Autodesk Fusion 360 part; units mm, degrees
sketch "스케치1" plane through (0, 0, 0) normal (0, 1, 0) x (1, 0, 0)
  line L0 (10, -10) -> (-10, -10)
  line L1 (-10, -10) -> (-10, 10)
  line L2 (-10, 10) -> (10, 10)
  line L3 (10, 10) -> (10, -10)
  line L4 (10, -10) -> (-10, 10) construction
  line L5 (-10, -10) -> (10, 10) construction
  line L6 (10, 0) -> (10, -4.15)
  line L7 (3.3, 0) -> (3.3, 4.15)
  line L8 (3.3, 4.15) -> (10, 4.15)
  line L9 (10, 4.15) -> (10, -4.15)
  line L10 (10, -4.15) -> (3.3, -4.15)
  line L11 (3.3, -4.15) -> (3.3, 4.15)
  line L12 (10, -4.15) -> (8.5, -4.15)
  line L13 (8.5, -4.15) -> (8.5, -2.65)
  line L14 (8.5, -2.65) -> (10, -2.65)
  line L15 (10, -2.65) -> (10, -4.15)
  line L16 (10, 4.15) -> (8.5, 4.15)
  line L17 (8.5, 4.15) -> (8.5, 2.65)
  line L18 (8.5, 2.65) -> (10, 2.65)
  line L19 (10, 2.65) -> (10, 4.15)
  line L20 (8.5, 4.15) -> (5.5, 4.15)
  line L21 (5.5, 4.15) -> (5.5, -4.15)
  line L22 (5.5, -4.15) -> (8.5, -4.15)
  line L23 (8.5, -4.15) -> (8.5, 4.15)
  spline S0 degree 5 poles (5.5, -4.15) (5.3331, -3.984) (5.014, -3.652) (4.579, -3.154) (4.0878, -2.49) (3.6321, -1.66) (3.3486, -0.83) (3.2516, 0) (3.3486, 0.83) (3.6321, 1.66) (4.0878, 2.49) (4.579, 3.154) (5.014, 3.652) (5.3331, 3.984) (5.5, 4.15) knots 0 0 0 0 0 0 0.1 0.2 0.3 0.4 0.5 0.6 0.7 0.8 0.9 1 1 1 1 1 1
  spline S1 degree 5 poles (4.15, 5.5) (3.984, 5.3331) (3.652, 5.014) (3.154, 4.579) (2.49, 4.0878) (1.66, 3.6321) (0.83, 3.3486) (0, 3.2516) (-0.83, 3.3486) (-1.66, 3.6321) (-2.49, 4.0878) (-3.154, 4.579) (-3.652, 5.014) (-3.984, 5.3331) (-4.15, 5.5) knots 0 0 0 0 0 0 0.1 0.2 0.3 0.4 0.5 0.6 0.7 0.8 0.9 1 1 1 1 1 1
  line L24 (4.15, 5.5) -> (4.15, 8.5)
  line L25 (4.15, 8.5) -> (2.65, 8.5)
  line L26 (2.65, 8.5) -> (2.65, 10)
  line L27 (-4.15, 8.5) -> (-4.15, 5.5)
  line L28 (-4.15, 8.5) -> (-2.65, 8.5)
  line L29 (-2.65, 8.5) -> (-2.65, 10)
  spline S2 degree 5 poles (-5.5, 4.15) (-5.3331, 3.984) (-5.014, 3.652) (-4.579, 3.154) (-4.0878, 2.49) (-3.6321, 1.66) (-3.3486, 0.83) (-3.2516, 0) (-3.3486, -0.83) (-3.6321, -1.66) (-4.0878, -2.49) (-4.579, -3.154) (-5.014, -3.652) (-5.3331, -3.984) (-5.5, -4.15) knots 0 0 0 0 0 0 0.1 0.2 0.3 0.4 0.5 0.6 0.7 0.8 0.9 1 1 1 1 1 1
  line L30 (-5.5, 4.15) -> (-8.5, 4.15)
  line L31 (-8.5, 4.15) -> (-8.5, 2.65)
  line L32 (-8.5, 2.65) -> (-10, 2.65)
  line L33 (-8.5, -4.15) -> (-5.5, -4.15)
  line L34 (-8.5, -4.15) -> (-8.5, -2.65)
  line L35 (-8.5, -2.65) -> (-10, -2.65)
  spline S3 degree 5 poles (-4.15, -5.5) (-3.984, -5.3331) (-3.652, -5.014) (-3.154, -4.579) (-2.49, -4.0878) (-1.66, -3.6321) (-0.83, -3.3486) (0, -3.2516) (0.83, -3.3486) (1.66, -3.6321) (2.49, -4.0878) (3.154, -4.579) (3.652, -5.014) (3.984, -5.3331) (4.15, -5.5) knots 0 0 0 0 0 0 0.1 0.2 0.3 0.4 0.5 0.6 0.7 0.8 0.9 1 1 1 1 1 1
  line L36 (-4.15, -5.5) -> (-4.15, -8.5)
  line L37 (-4.15, -8.5) -> (-2.65, -8.5)
  line L38 (-2.65, -8.5) -> (-2.65, -10)
  line L39 (4.15, -8.5) -> (4.15, -5.5)
  line L40 (4.15, -8.5) -> (2.65, -8.5)
  line L41 (2.65, -8.5) -> (2.65, -10)
  line L42 (-10, -10) -> (-4.15, -10)
  line L43 (-4.15, -10) -> (-4.15, -4.15)
  line L44 (-4.15, -4.15) -> (-10, -4.15)
  line L45 (-10, -4.15) -> (-10, -10)
  circle A0 centre (-7.075, -7.075) radius 2
  circle A1 centre (7.075, -7.075) radius 2
  circle A2 centre (7.075, 7.075) radius 2
  circle A3 centre (-7.075, 7.075) radius 2
  point P0 (0, 3.3)
  point P1 (-3.3, 0)
  point P2 (0, -3.3)
  dimension "d1" = 20
  dimension "d2" = 20
  dimension "d3" = 6.7
  dimension "d4" = 4.15
  dimension "d5" = 4.15
  dimension "d6" = 1.5
  dimension "d7" = 1.5
  dimension "d8" = 1.5
  dimension "d9" = 1.5
  dimension "d10" = 3
  dimension "d12" = 360
  dimension "d13" = 5.85
  dimension "d14" = 4
  dimension "d16" = 360
extrude "돌출1" add sketch "스케치1" along normal blind 50 contours L0 L1 L2 L3 L7 L8 L10 L11 L12 L16 L20 L22 S1 L24 L25 L26 L27 L28 L29 S2 L30 L31 L32 S3 L39 L40 L41 L43 L44 | L3 L6 L9 L10 L12 L13 L14 L15 L23 | L0 L37 L38 L43 | L0 L1 L33 L36 L42 L43 L44 L45 | L10 L11 S0 | L3 L8 L9 L16 L17 L18 L19 L23 | L7 L8 L11 S0 | L1 L34 L35 L44
Work out the finished part from the listing and answer in its coordinate system (mm). A direction names the side the tool comes from. Give positions to 0.01 mm unless a question says otherwise; leave off trailing zeros. Loops run counter-clockwise (first coordinate to the right, second up) from the corner with the lowest first, then second, coordinate; pieces in that order, holes last. Notation, with made-up numbers: (39.5, -38) -> (87.5, -38) arc R26 ccw to (87.5, -23) -> close; hole circle Ø2 at (15.5, 9). An arc over 180 degrees is marked (long way). Use a Markdown table: item, result. Add a question column.
1) Which of the six approach directions +Z, -Z, +X, -X, +Y, -Y give full straight-line access (tool end or side, diameter ignored) to faces 4 (the flat face through (-10, 25, -6)), 5 (the flat face through (3, 25, 8.5)), 6 (the flat face through (-2.65, 25, 9))?
2) For a pull along X with two mould halves and no side action, classify faces 1 (the flat face through (-9, 25, -2.65)), 2 (the flat face through (10, 25, 6)), 3 (the flat face through (4.15, 25, -7)) as +X half, -X half, draft (parallel to the pull), parting line (faces both ways), or undercut.
3) The part is cut by section A-A, the plane x = 6.75. Determine the outline of the cut face in (y, z), plus the area to 3 significant figures.
4) The part is cut by section B-B, the plane y = 5. Count the separate pieces of the cut face and the enclosed holes in it, plus the area to 3 significant figures.
5) Consider line 1 along Z through (x, y) = (7, 16); line 2 along Z through (x, y) = (-5.75, 19.5); line 3 along X through (y, z) = (39, -4). Determine where each line is inside the solid, lowest interval first.
6) Each of these flat-tipped pins is pushed along its axis until it touches: P1, Ø2, axis at x = 0.5, z = 6.5, coming from the -Y side; P2, Ø3, axis at x = 1, y = 31, coming from the +Z side; P3, Ø4, axis at x = 0, y = 22.5, coming from the +Z side. Where does it stop, or does it pass through?
Reported:
| question | item | result |
|---|---|---|
| 1 | face 4 | +Z, -Z, -X, +Y, -Y |
| 1 | face 5 | +Y, -Y |
| 1 | face 6 | +Z, +Y, -Y |
| 2 | face 1 | draft |
| 2 | face 2 | +X half |
| 2 | face 3 | undercut |
| 3 | outline | (0, -10) -> (50, -10) -> (50, -9.05) -> (0, -9.05) -> close; (0, -5.1) -> (50, -5.1) -> (50, -4.15) -> (0, -4.15) -> close; (0, 4.15) -> (50, 4.15) -> (50, 5.1) -> (0, 5.1) -> close; (0, 9.05) -> (50, 9.05) -> (50, 10) -> (0, 10) -> close |
| 3 | area | 190 mm^2 |
| 4 | separate pieces | 1 |
| 4 | enclosed holes | 4 |
| 4 | area | 170 mm^2 |
| 5 | line 1 | z = -10 to -9.07, -5.08 to -4.15, 4.15 to 5.08, 9.07 to 10 |
| 5 | line 2 | z = -10 to -8.57, -5.58 to -4.15, 4.15 to 5.58, 8.57 to 10 |
| 5 | line 3 | x = -10 to -8.5, -5.35 to -2.28, 2.28 to 5.35, 8.5 to 10 |
| 6 | P1 | passes through |
| 6 | P2 | stops at z = 4.13 |
| 6 | P3 | stops at z = 3.84 |
